from build123d import *

# Parameters (mm, degrees)
SKETCH1_W           = 30
SKETCH1_H           = 5
BOSS_EXTRUDE1_START = 15
BOSS_EXTRUDE1_DEPTH = 0.5
BOSS_EXTRUDE2_START = -15.5
BOSS_EXTRUDE2_DEPTH = 0.5


with BuildPart() as part:
    # Sketch1 → Revolve1 (revolve)
    with BuildSketch(Plane(origin=(0, 0, 0), x_dir=(0, 0, -1), z_dir=(1, 0, 0)), mode=Mode.PRIVATE) as revolve1_sk:
        with Locations((0, 2.5)):
            Rectangle(SKETCH1_W, SKETCH1_H)
    revolve(revolve1_sk.sketch.rotate(Axis((0, 0, 15), (0, 0, -1)), 90), axis=Axis((0, 0, 15), (0, 0, -1)))

    # Sketch2 → Boss-Extrude1 (add)
    with BuildSketch(Plane.XY.offset(BOSS_EXTRUDE1_START)):
        with BuildLine():
            Line((-13, -2.5), (0, -2.5))
            ThreePointArc((0, -2.5), (2.5, 0), (0, 2.5))
            Line((0, 2.5), (-13, 2.5))
            Line((-13, 2.5), (-13, -2.5))
        make_face()
    extrude(amount=BOSS_EXTRUDE1_DEPTH)

    # Sketch2<2> → Boss-Extrude2 (add)
    with BuildSketch(Plane.XY.offset(BOSS_EXTRUDE2_START)):
        with BuildLine():
            Line((-13, -2.5), (0, -2.5))
            ThreePointArc((0, -2.5), (2.5, 0), (0, 2.5))
            Line((0, 2.5), (-13, 2.5))
            Line((-13, 2.5), (-13, -2.5))
        make_face()
    extrude(amount=BOSS_EXTRUDE2_DEPTH)


solid = part.part
The model under review builds one solid part; all positions refer to its coordinate system, in mm. A direction names the side the tool comes from. Round coordinates to 2 decimals unless told otherwise and drop trailing zeros. Order: outer loops, then holes, each group sorted by start corner. A loop starts at its lowest first (then second) coordinate and runs counter-clockwise, first axis right, second up. Notation, with made-up numbers: (61.5, 21) - (120.5, 21) arc R6 ccw to (120.5, 27) - close; hole circle Ø2 at (76.25, -9.75). An arc over 180 degrees is marked (long way). Use one line per item in the form item = value.
Q1. Tool access review of faces 5 (the cylindrical face through (2.5, -0.1, -15.3)), 6 (the flat face through (-5, 0, 15.5)): name each direction out of +Z, -Z, +X, -X, +Y, -Y from which nothing blocks a thin tool from reaching the whole face with its end or side.
Response values:
face_5 = -Z, +X
face_6 = +Z, +X, -X, +Y, -Y
Q2. Add section A-A on x = -9.5. Give the boundary of the cut face in (y, z), then the cut area to 3 significant figures.
Response values:
outline = (-2.5, -15.5) - (2.5, -15.5) - (2.5, -15) - (-2.5, -15) - close; (-2.5, 15) - (2.5, 15) - (2.5, 15.5) - (-2.5, 15.5) - close
area = 5.00 mm^2
Q3. Clearance check with a flat-ended pin moving along its axis: P1, Ø0.6, axis at x = -5, z = -15.5, coming from the -Y side. State where the tip first meets the part, or that it passes through.
Response values:
P1 = -2.5
Q4. Add section D-D on y = 1.5. Give the boundary of the cut face in (x, z), then the cut area to 3 significant figures.
Response values:
outline = (-13, -15.5) - (2, -15.5) - (2, -15) - (4.77, -15) - (4.77, 15) - (2, 15) - (2, 15.5) - (-13, 15.5) - (-13, 15) - (-4.77, 15) - (-4.77, -15) - (-13, -15) - close
area = 301 mm^2
Q5. Add section B-B on y = 0. Give the boundary of the cut face in (x, z), then the cut area to 4 significant figures.
Response values:
outline = (-13, -15.5) - (2.5, -15.5) - (2.5, -15) - (5, -15) - (5, 15) - (2.5, 15) - (2.5, 15.5) - (-13, 15.5) - (-13, 15) - (-5, 15) - (-5, -15) - (-13, -15) - close
area = 315.5 mm^2
Q6. Add section C-C on z = -3.5. Give the boundary of the cut face in (x, y), then the cut area to 3 significant figures.
Response values:
outline = circle Ø10 at (0, 0)
area = 78.5 mm^2
Q7. To check wall thickness, follow line 1 (Z direction, x = -9, y = -0.5); line 2 (Z direction, x = 2.75, y = -0.5); line 3 (X direction, y = -0.75, z = -13). State the ranges of each line that lie inside material, in increasing order.
Response values:
line_1 = -15.5 to -15, 15 to 15.5
line_2 = -15 to 15
line_3 = -4.94 to 4.94
Q8. Mouldability with a two-part tool opening along Z and no side actions: class faces 1 (the cylindrical face through (2.5, -0.1, 15.2)), 2 (the flat face through (-9, 0, 15)), 3 (the flat face through (2.5, 1, 15)), 4 (the flat face through (-9, 0, -15)) as pulls with the +Z half, pulls with the -Z half, needs draft (parallel to the pull), parting line crosses it, or undercut.
Response values:
face_1 = needs draft
face_2 = undercut
face_3 = pulls with the +Z half
face_4 = undercut
